Autodesk Inventor part; units mm, degrees
ref_plane "YZ Plane" through (0, 0, 0) normal (1, 0, 0) x (0, 1, 0)
ref_plane "XZ Plane" through (0, 0, 0) normal (0, 1, 0) x (-1, 0, 0)
ref_plane "XY Plane" through (0, 0, 0) normal (0, 0, 1) x (1, 0, 0)
sketch "スケッチ1" plane through (0, 0, 0) normal (0, 1, 0) x (-1, 0, 0)
  circle A0 centre (0, 0) radius 3.15
  dimension "d0" = 6.3
extrude "押し出し1" add sketch "スケッチ1" along normal blind 1.5
sketch "スケッチ2" plane through (0, 0, 0) normal (0, -1, 0) x (1, 0, 0)
  circle A0 centre (0, 0) radius 2.1
  dimension "d3" = 4.2
extrude "押し出し2" add sketch "スケッチ2" along normal blind 0.77
sketch "スケッチ3" plane through (0, 1.5, 0) normal (0, 1, 0) x (1, 0, 0)
  point P0 (0, 0)
  point P1 (0, 0)
hole "穴1" at (0, 1.5, 0) direction (0, -1, 0) diameter 3 end through all
thread "ねじ1"
fillet "フィレット1" radius 0.3 1 edges at (3.15, 1.5, 0)
fillet "フィレット1" radius 0.1 1 edges at (3.15, 0, 0)
sketch "スケッチ4" plane through (0, 0, 0) normal (1, 0, 0) x (0, 1, 0)
  line L0 (-0.77, 2.1) -> (-0.77, -2.1)
  line L1 (-0.77, 2.1) -> (-0.37, 1.9)
  line L2 (-0.37, 1.9) -> (-0.37, 2.1)
  line L3 (-0.37, 2.1) -> (-0.77, 2.1)
  line L4 (-1.956, 0) -> (2.076, 0)
  point P0 (0, 0)
  dimension "d17" = 0.4
  dimension "d18" = 0.2
revolve "回転1" cut sketch "スケッチ4" angle 360 about axis through (0, -10, 0) along (0, 1, 0)
properties part number "ClinchingNut_M3T1.5_Slab0.8"
CAD build for the part. Positions are in the model's coordinates, mm. A direction names the side the tool comes from. Coordinates: 2 decimals unless noted, no trailing zeros. Write each loop counter-clockwise with the first axis right and the second up, starting at its lowest first coordinate (ties: lowest second). Pieces come first, ordered by that corner, then holes. Notation, with made-up numbers: (29, -6.5) - (54, -6.5) arc R22 cw to (54, 32.5) - close; hole circle Ø10 at (29.25, 71). An arc over 180 degrees is marked (long way). Use a Markdown table: item, result. Add a question column.
Item 1: 3-axis set-ups, long thin cutter, end or side, ignore diameter. For faces 1 (the face through (2.5, 0.642, 1.917)), 2 (the face through (2.003, -0.182, -0.631)): which of +Z, -Z, +X, -X, +Y, -Y reach the whole face in a straight line?
Item 2: Drill centre lines: L1, parallel to X at y = -0.05, z = 0; L2, parallel to Z at x = 0, y = 0.7. Where is each one in solid material? Low to high. Write a range as from..to.
Item 3: Flat gauge pin, fed straight in: pin 1 (1 mm diameter, centred on x = -1, y = 1, fed in from +Z). Where does the tip first touch, or does it go through?
Item 4: Band-saw the part on C-C, the plane y = 0.9. Give the cut face in (x, z).
Item 5: Band-saw the part on B-B, the plane x = 0. Give the cut face in (y, z), and give its area (3 significant figures).
Item 6: Band-saw the part on A-A, the plane z = 0. Give the cut face in (x, y), and give its area (3 significant figures).
Item 7: Band-saw the part on D-D, the plane y = -0.1. Give the cut face in (x, z), and give its area (3 significant figures).
Numbers:
| question | item | result |
|---|---|---|
| 1 | face 1 | +Y, -Y |
| 1 | face 2 | -Y |
| 2 | L1 | -2.1..-1.5, 1.5..2.1 |
| 2 | L2 | -3.15..-1.5, 1.5..3.15 |
| 3 | pin 1 | z = 3.11 |
| 4 | outline | circle Ø6.3 at (0, 0); hole circle Ø3 at (0, 0) |
| 5 | outline | (-0.77, -2.1) - (-0.37, -1.9) - (-0.37, -2.1) - (0, -2.1) - (0, -3.05) arc R0.1 ccw to (0.1, -3.15) - (1.2, -3.15) arc R0.3 ccw to (1.5, -2.85) - (1.5, -1.5) - (-0.77, -1.5) - close; (-0.77, 1.5) - (1.5, 1.5) - (1.5, 2.85) arc R0.3 ccw to (1.2, 3.15) - (0.1, 3.15) arc R0.1 ccw to (0, 3.05) - (0, 2.1) - (-0.37, 2.1) - (-0.37, 1.9) - (-0.77, 2.1) - close |
| 5 | area | 5.75 mm2 |
| 6 | outline | (-3.15, 0.1) arc R0.1 ccw to (-3.05, 0) - (-2.1, 0) - (-2.1, -0.37) - (-1.9, -0.37) - (-2.1, -0.77) - (-1.5, -0.77) - (-1.5, 1.5) - (-2.85, 1.5) arc R0.3 ccw to (-3.15, 1.2) - close; (1.5, -0.77) - (2.1, -0.77) - (1.9, -0.37) - (2.1, -0.37) - (2.1, 0) - (3.05, 0) arc R0.1 ccw to (3.15, 0.1) - (3.15, 1.2) arc R0.3 ccw to (2.85, 1.5) - (1.5, 1.5) - close |
| 6 | area | 5.75 mm2 |
| 7 | outline | circle Ø4.2 at (0, 0); hole circle Ø3 at (0, 0) |
| 7 | area | 6.79 mm2 |
